The drawing under review shows one solid part. Ordinate dimensions are in mm from its lowest x, y, z. A direction names the side the tool comes from. Give positions to 0.01 mm unless a question says otherwise; leave off trailing zeros. Order: outer loops, then holes, each group sorted by start corner. A loop starts at its lowest first (then second) coordinate and runs counter-clockwise, first axis right, second up. Notation, with made-up numbers: (54, 88) - (110, 88) arc R15 ccw to (110, 93) - close; hole circle Ø7 at (-0.5, 57). An arc over 180 degrees is marked (long way). Use CSV: the item, a comma, the result in double quotes.
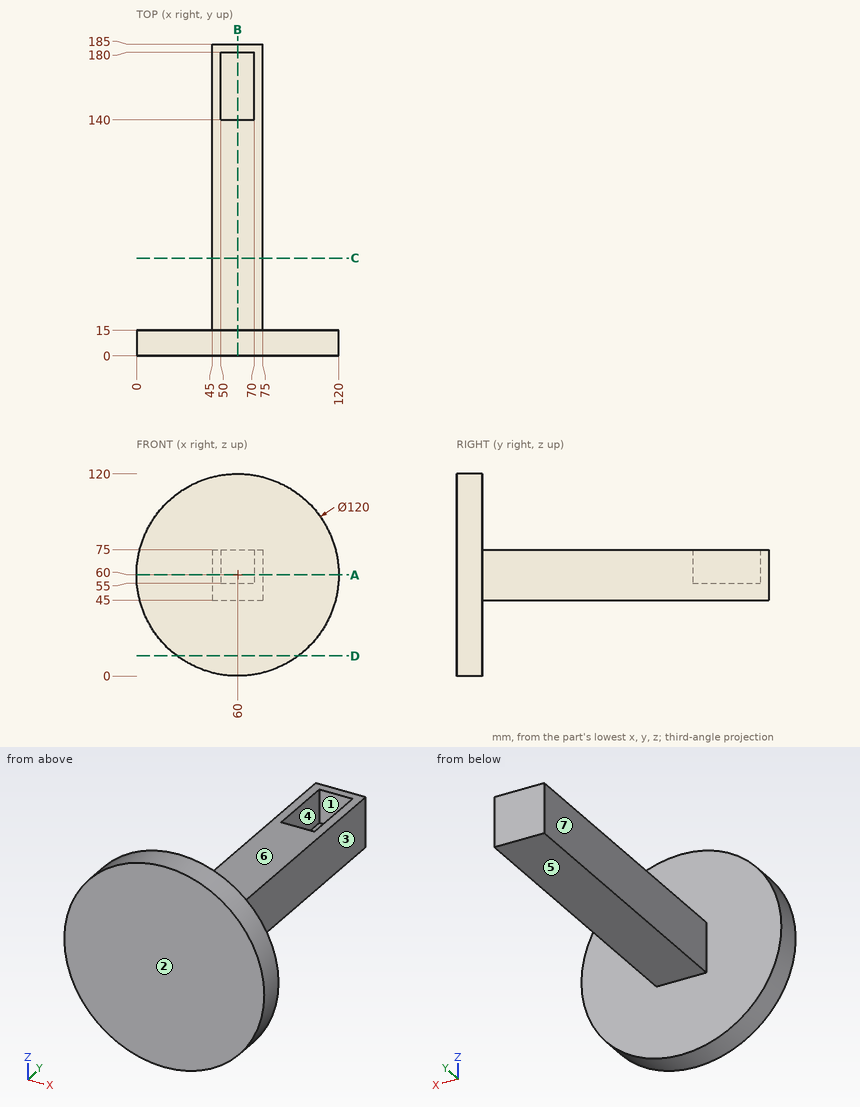
Item 1: Clearance check with flat-ended pins moving along their axes: pin 1 (24 mm diameter, centred on x = 60.5, y = 111, fed in from +Z); pin 2 (4 mm diameter, centred on x = 67.5, z = 98.5, fed in from +Y); pin 3 (10 mm diameter, centred on y = 160.5, z = 70, fed in from +X). State where each tip first meets the part, or that it passes through.
Results list:
pin 1,"stops at z = 75"
pin 2,"stops at y = 15"
pin 3,"stops at x = 75"
Item 2: Take a section at C-C, the plane y = 58. Give the boundary of the cut face in (x, z), and give its area (3 significant figures).
Results list:
outline,"(45, 45) - (75, 45) - (75, 75) - (45, 75) - close"
area,"900 mm2"
Item 3: Take a section at A-A, the plane z = 60. Give the boundary of the cut face in (x, y), and give its area (3 significant figures).
Results list:
outline,"(0, 0) - (120, 0) - (120, 15) - (75, 15) - (75, 185) - (45, 185) - (45, 15) - (0, 15) - close; hole (50, 140) - (70, 140) - (70, 180) - (50, 180) - close"
area,"6,100 mm2"
Item 4: Mouldability with a two-part tool opening along Y and no side actions: class the marked faces 1, 2 and 3 as pulls with the +Y half, pulls with the -Y half, needs draft (parallel to the pull), parting line crosses it, or undercut.
Results list:
face 1,"undercut"
face 2,"pulls with the -Y half"
face 3,"needs draft"
Item 5: Take a section at B-B, the plane x = 60. Give the boundary of the cut face in (y, z).
Results list:
outline,"(0, 0) - (15, 0) - (15, 45) - (185, 45) - (185, 75) - (180, 75) - (180, 55) - (140, 55) - (140, 75) - (15, 75) - (15, 120) - (0, 120) - close"
Item 6: Take a section at D-D, the plane z = 12. Give the boundary of the cut face in (x, y), and give its area (3 significant figures).
Results list:
outline,"(24, 0) - (96, 0) - (96, 15) - (24, 15) - close"
area,"1,080 mm2"
Item 7: Tool access review of the marked faces 4, 5, 6 and 7: name each direction out of +Z, -Z, +X, -X, +Y, -Y from which nothing blocks a thin tool from reaching the whole face with its end or side.
Results list:
face 4,"+Z"
face 5,"-Z, +X, -X, +Y"
face 6,"+Z, +X, -X, +Y"
face 7,"+Z, -Z, -X, +Y"
Item 8: Wall thickness on L1, parallel to Y at x = 60, z = 5; L2, parallel to X at y = 74.5, z = 46.5: over which ranges is each line inside the solid? List them lowest first.
Results list:
L1,"y = 0 to 15"
L2,"x = 45 to 75"
